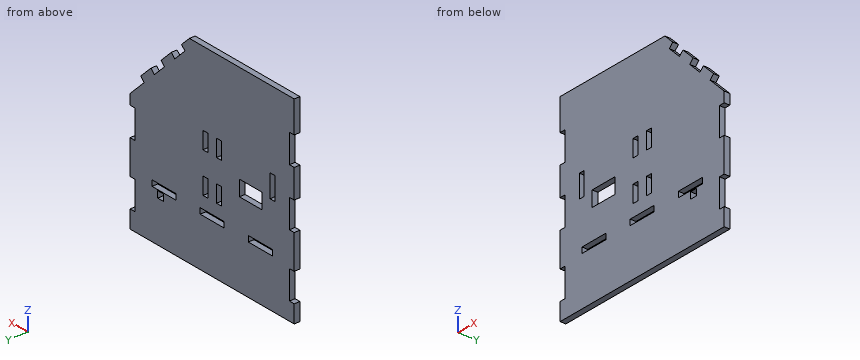
```python
from build123d import *

# Parameters (mm, degrees)
SKETCH_W   = 49.6
SKETCH_H   = 10
SKETCH_W_2 = 10
SKETCH_H_2 = 39.8
SKETCH_W_3 = 47
SKETCH_H_3 = 27
SKETCH_H_4 = 29.8
SKETCH_W_4 = 12.5
SKETCH_H_5 = 11.5
PAD_DEPTH  = 10


with BuildPart() as part:
    # Sketch → Pad (new body)
    with BuildSketch(Plane.XZ):
        Polygon((0, 0), (0, 30.933), (10, 30.933), (10, 80.733), (0, 80.733), (0, 140.2), (10, 140.2), (10, 190), (0, 190), (0, 240), (10, 240), (10, 289.8), (0, 289.8), (0, 345), (217.0709, 345), (233.405067, 328.665833), (226.333999, 321.594766), (247.405781, 300.522983), (254.476849, 307.594051), (275.690052, 286.380848), (268.618985, 279.30978), (289.690767, 258.237998), (296.761835, 265.309066), (317.975038, 244.095862), (310.90397, 237.024795), (340, 207.928765), (340, 189.999765), (330, 189.999765), (330, 140.199765), (340, 140.199765), (340, 80.733), (330, 80.733), (330, 30.933), (340, 30.933), (340, 0), align=None)
        with Locations((70.2, 90)):
            Rectangle(SKETCH_W, SKETCH_H, mode=Mode.SUBTRACT)
        with Locations((170, 90)):
            Rectangle(SKETCH_W, SKETCH_H, mode=Mode.SUBTRACT)
        with Locations((269.8, 90)):
            Rectangle(SKETCH_W, SKETCH_H, mode=Mode.SUBTRACT)
        with Locations((45, 190.5)):
            Rectangle(SKETCH_W_2, SKETCH_H_2, mode=Mode.SUBTRACT)
        with Locations((90, 160)):
            Rectangle(SKETCH_W_3, SKETCH_H_3, mode=Mode.SUBTRACT)
        with Locations((156, 201.16)):
            Rectangle(SKETCH_W_2, SKETCH_H_4, mode=Mode.SUBTRACT)
        with Locations((184, 201.16)):
            Rectangle(SKETCH_W_2, SKETCH_H_4, mode=Mode.SUBTRACT)
        with Locations((156, 131.16)):
            Rectangle(SKETCH_W_2, SKETCH_H_4, mode=Mode.SUBTRACT)
        with Locations((184, 131.16)):
            Rectangle(SKETCH_W_2, SKETCH_H_4, mode=Mode.SUBTRACT)
        with Locations((276.54, 77.73)):
            Rectangle(SKETCH_W_4, SKETCH_H_5, mode=Mode.SUBTRACT)
    extrude(amount=PAD_DEPTH)


solid = part.part
```
Check sheet for the modelled part. Datum: model origin and axes. Units: mm. Coordinates: 2 decimals unless noted, no trailing zeros. Write each loop counter-clockwise with the first axis right and the second up, starting at its lowest first coordinate (ties: lowest second). Pieces come first, ordered by that corner, then holes. Notation, with made-up numbers: M -22,-34.5 L 21,-34.5 A22 cw 21,1.5 Z; hole C 48.25,-4 d9. An arc over 180 degrees is marked long. Write item = value, one per line. Start each with the question number.
1. Sectioned sample at B-B (x = 105). Record the cut outline in (y, z).
2. Sectioned sample at D-D (z = 55). Record the cut outline in (x, y).
3. Go/stop test with flat-tipped pins: pin 1 (3 mm diameter, centred on y = -6, z = 182.5, fed in from +X); pin 2 (3 mm diameter, centred on y = -6, z = 268, fed in from -X). Record where each tip stops, or that it passes through.
4. Sectioned sample at C-C (y = -1.5). State how many separate pieces and enclosed holes the cut face has, then the cut area to 3 significant figures.
5. Sectioned sample at A-A (x = 155.5). Record the cut outline in (y, z), then the cut area to 3 significant figures.
6. Thickness scan on probe 1 along X at (y, z) = (-2.5, 122); probe 2 along Z at (x, y) = (79.5, -2.75); probe 3 along X at (y, z) = (-3.5, 195.5). Record the ranges inside material, lowest first.
The answers:
q1.outline = M -10,0 L 0,0 L 0,146.5 L -10,146.5 Z; M -10,173.5 L 0,173.5 L 0,345 L -10,345 Z
q2.outline = M 10,-10 L 330,-10 L 330,0 L 10,0 Z
q3.pin_1 = 330
q3.pin_2 = 10
q4.separate_pieces = 1
q4.enclosed_holes = 10
q4.area = 102,000 mm²
q5.outline = M -10,0 L 0,0 L 0,85 L -10,85 Z; M -10,95 L 0,95 L 0,116.26 L -10,116.26 Z; M -10,146.06 L 0,146.06 L 0,186.26 L -10,186.26 Z; M -10,216.06 L 0,216.06 L 0,345 L -10,345 Z
q5.area = 2,750 mm²
q6.probe_1 = 0 to 151, 161 to 179, 189 to 340
q6.probe_2 = 0 to 85, 95 to 146.5, 173.5 to 345
q6.probe_3 = 0 to 40, 50 to 151, 161 to 179, 189 to 340
